```python
from build123d import *

# Parameters (mm, degrees)
F0_W     = 50.8
F0_H     = 50.8
F1_DEPTH = 50.8
F2_R     = 12.7
F3_DEPTH = 50.8
F4_W     = 25.4
F4_H     = 25.4
F5_DEPTH = 12.7
F6_R     = 17.614726
F7_DEPTH = 12.7


with BuildPart() as f1:
    # F0 (on Front) → F1 (new body)
    with BuildSketch(Plane.XZ):
        with Locations((-17.660277, -1.05328)):
            Rectangle(F0_W, F0_H)
    extrude(amount=F1_DEPTH)

    # F2 (on face) → F3 (cut)
    with BuildSketch(Plane.XY.offset(24.34672)):
        with Locations((-16.899487, -27.783902)):
            Circle(F2_R)
    extrude(amount=-F3_DEPTH, mode=Mode.SUBTRACT)

    # F4 (on Right) → F5 (join)
    with BuildSketch(Plane.YZ):
        with Locations((-22.722087, -2.098986)):
            Rectangle(F4_W, F4_H)
    extrude(amount=F5_DEPTH)

    # F6 (on face) → F7 (join)
    with BuildSketch(Plane.XZ.offset(50.8)):
        with Locations((-18.427124, 0)):
            Circle(F6_R)
    extrude(amount=F7_DEPTH)


solid = f1.part
```
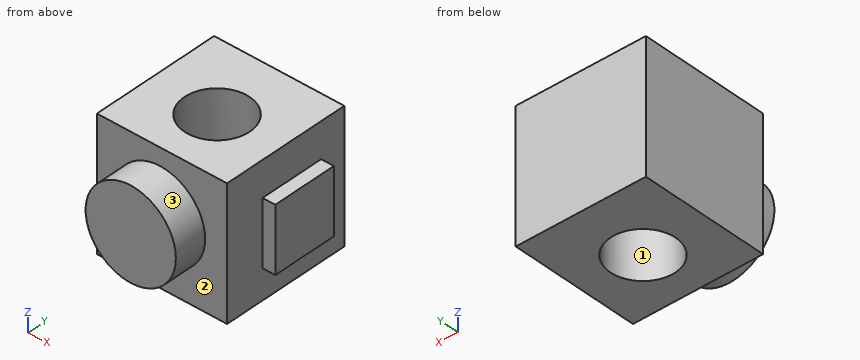
Design review of the part built by this model. Coordinates are the model's own, in mm. Face numbers are marked on the shaded views. Coordinates: 2 decimals unless noted, no trailing zeros. Order: outer loops, then holes, each group sorted by start corner. A loop starts at its lowest first (then second) coordinate and runs counter-clockwise, first axis right, second up. Notation, with made-up numbers: M 74,-25 L 107,-25 A18 ccw 107,-12 Z; hole C 16,4 d9. An arc over 180 degrees is marked long. Answer as a JSON object with one key per item and string values. Group by question number.
1) Wall thickness on L1, parallel to Y at x = -17, z = -20; L2, parallel to X at y = -49, z = 6.5; L3, parallel to Y at x = -28, z = 3: over which ranges is each line inside the solid? List them lowest first.
2) Add section D-D, the plane y = -5. Write out the cut boundary in (x, z).
3) For pin 1 (4 mm diameter, centred on x = 10, z = -8.5, fed in from +Y); pin 2 (1.5 mm diameter, centred on x = 10.5, z = 1, fed in from -Y); pin 3 (3 mm diameter, centred on x = -29.5, z = -8.5, fed in from +Y); pin 4 (8 mm diameter, centred on y = -43, z = -21, fed in from +X), all flat-tipped, find the tip position at first contact; note any pin that passes through.
4) Add section B-B, the plane z = 13.5. Write out the cut boundary in (x, y), then the cut area to 3 significant figures.
5) Add section A-A, the plane x = -13. Write out the cut boundary in (y, z).
6) Add section C-C, the plane x = -25. Write out the cut boundary in (y, z), then the cut area to 3 significant figures.
7) Mouldability with a two-part tool opening along X and no side actions: class the marked faces 1, 2 and 3 as pulls with the +X half, pulls with the -X half, needs draft (parallel to the pull), parting line crosses it, or undercut.
Computed values:
{
 "1": {"L1": "y = -50.8 to -40.48, -15.08 to 0", "L2": "x = -43.06 to 7.74", "L3": "y = -63.5 to -33.95, -21.61 to 0"},
 "2": {"outline": "M -43.06,-26.45 L 7.74,-26.45 L 7.74,24.35 L -43.06,24.35 Z"},
 "3": {"pin 1": "stops at y = -10.02", "pin 2": "stops at y = -35.42", "pin 3": "stops at y = 0", "pin 4": "stops at x = 7.74"},
 "4": {"outline": "M -43.06,-50.8 L -29.74,-50.8 L -29.74,-63.5 L -7.11,-63.5 L -7.11,-50.8 L 7.74,-50.8 L 7.74,0 L -43.06,0 Z; hole C -16.9,-27.78 d25.4", "area": "2,360 mm^2"},
 "5": {"outline": "M -63.5,-16.76 L -50.8,-16.76 L -50.8,-26.45 L -39.87,-26.45 L -39.87,24.35 L -50.8,24.35 L -50.8,16.76 L -63.5,16.76 Z; M -15.7,-26.45 L 0,-26.45 L 0,24.35 L -15.7,24.35 Z"},
 "6": {"outline": "M -63.5,-16.34 L -50.8,-16.34 L -50.8,-26.45 L -37.57,-26.45 L -37.57,24.35 L -50.8,24.35 L -50.8,16.34 L -63.5,16.34 Z; M -18,-26.45 L 0,-26.45 L 0,24.35 L -18,24.35 Z", "area": "2,000 mm^2"},
 "7": {"face 1": "undercut", "face 2": "needs draft", "face 3": "parting line crosses it"}
}
